```python
from build123d import *

# Parameters (mm, degrees)
ESQUISSE1_W             = 385
ESQUISSE1_H             = 40
BOSS_EXTRU_1_DEPTH      = 6
ESQUISSE3_W             = 100
ESQUISSE3_H             = 6
BOSS_EXTRU_2_DEPTH      = 6
ENL_V_MAT_EXTRU_1_DEPTH = 47


with BuildPart() as part:
    # Esquisse1 → Boss.-Extru.1 (new body)
    with BuildSketch(Plane.XY):
        Rectangle(ESQUISSE1_W, ESQUISSE1_H)
    extrude(amount=BOSS_EXTRU_1_DEPTH)

    # Esquisse3 → Boss.-Extru.2 (add)
    with BuildSketch(Plane.XY.offset(6)):
        with Locations((-92.5, 23)):
            Rectangle(ESQUISSE3_W, ESQUISSE3_H)
        with Locations((92.5, 23)):
            Rectangle(ESQUISSE3_W, ESQUISSE3_H)
        with Locations((92.5, -23)):
            Rectangle(ESQUISSE3_W, ESQUISSE3_H)
        with Locations((-92.5, -23)):
            Rectangle(ESQUISSE3_W, ESQUISSE3_H)
    extrude(amount=-BOSS_EXTRU_2_DEPTH)

    # Esquisse4 → Enlèv. mat.-Extru.1 (cut, through all)
    with BuildSketch(Plane(origin=(0, 20, 0), x_dir=(1, 0, 0), z_dir=(0, 1, 0))):
        Polygon((-192.5, -6), (-167.5, 0), (-192.5, 0), align=None)
        Polygon((192.5, -6), (167.5, 0), (192.5, 0), align=None)
    extrude(amount=-ENL_V_MAT_EXTRU_1_DEPTH, mode=Mode.SUBTRACT)


solid = part.part
```
The model under review builds one solid part; all positions refer to its coordinate system, in mm. A direction names the side the tool comes from. Round coordinates to 2 decimals unless told otherwise and drop trailing zeros. Order: outer loops, then holes, each group sorted by start corner. A loop starts at its lowest first (then second) coordinate and runs counter-clockwise, first axis right, second up.
Item 1: To check wall thickness, follow probe 1 along X at (y, z) = (23, 2.3); probe 2 along Y at (x, z) = (25.5, 1.65). State the ranges of each line that lie inside material, in increasing order.
Working result:
probe 1: x = -142.5 to -42.5, 42.5 to 142.5
probe 2: y = -20 to 20
Item 2: Add section C-C, the plane x = 24. State the section outline as (y, z) points.
Working result:
outline: (-20, 0) - (20, 0) - (20, 6) - (-20, 6) - close
Item 3: For pin 1 (1.8 mm diameter, centred on y = 21.5, z = 2.5, fed in from +X); pin 2 (1.8 mm diameter, centred on y = 23.5, z = 4.5, fed in from -X); pin 3 (8 mm diameter, centred on x = -127, y = -15, fed in from -Z); pin 4 (3 mm diameter, centred on x = -3.5, z = 3.5, fed in from +Y), all flat-tipped, find the tip position at first contact; note any pin that passes through.
Working result:
pin 1: stops at x = 142.5
pin 2: stops at x = -142.5
pin 3: stops at z = 0
pin 4: stops at y = 20
Item 4: Machinability: for faces 4 (the flat face through (-1, -20, 3)), 5 (the flat face through (142.5, -23, 3)), 6 (the flat face through (42.5, 23, 3)), 7 (the flat face through (-142.5, 23, 3)), 8 (the flat face through (162, 20, 3)), which of the approach directions +Z, -Z, +X, -X, +Y, -Y give a long, thin tool a straight path to every point of the face, cutting with its end or side? Answer none if there is none.
Working result:
face 4: +Z, -Z, -Y
face 5: +Z, -Z, +X, -Y
face 6: +Z, -Z, +Y
face 7: +Z, -Z, -X, +Y
face 8: +Z, -Z, +X, +Y
Item 5: Draft analysis for pull direction X (two halves, no side actions). For faces 1 (the flat face through (142.5, 23, 3)), 2 (the flat face through (-42.5, -23, 3)), 3 (the flat face through (-162, 20, 3)), state which applies: released by +X, released by -X, zero draft, split by the parting line, or undercut.
Working result:
face 1: released by +X
face 2: undercut
face 3: zero draft
Item 6: Add section B-B, the plane y = -14.5. State the section outline as (x, z) points.
Working result:
outline: (-192.5, 6) - (-167.5, 0) - (167.5, 0) - (192.5, 6) - close
Item 7: Add section A-A, the plane z = 1.2. State the section outline as (x, y) points.
Working result:
outline: (-172.5, -20) - (-142.5, -20) - (-142.5, -26) - (-42.5, -26) - (-42.5, -20) - (42.5, -20) - (42.5, -26) - (142.5, -26) - (142.5, -20) - (172.5, -20) - (172.5, 20) - (142.5, 20) - (142.5, 26) - (42.5, 26) - (42.5, 20) - (-42.5, 20) - (-42.5, 26) - (-142.5, 26) - (-142.5, 20) - (-172.5, 20) - close
